The listing builds one solid part. Answer for the finished solid, in the listing's coordinates (mm). A direction names the side the tool comes from. Coordinates: 2 decimals unless noted, no trailing zeros. Loops run counter-clockwise (first coordinate to the right, second up) from the corner with the lowest first, then second, coordinate; pieces in that order, holes last. Notation, with made-up numbers: M 59,84 L 67,84 A29 cw 67,112 Z; hole C 50.5,37.25 d1. An arc over 180 degrees is marked long. Return JSON: item names as keys, results as strings. Group by question number.
1. Which of the six approach directions +Z, -Z, +X, -X, +Y, -Y give full straight-line access (tool end or side, diameter ignored) to faces 4 (the face through (21, -15, 3)), 5 (the face through (10, -20, 3)), 6 (the face through (10, 20, 3))?
2. The mould has two halves that part along Y. Classify faces 1 (the face through (9.5, -16, 3)), 2 (the face through (34.71, 20.62, 2.96)), 3 (the face through (-0.5, -17, 3)): pulls with the +Y half, pulls with the -Y half, needs draft (parallel to the pull), parting line crosses it, or undercut.
3. Straight lines are drawn through the part: L1, parallel to Y at x = 20, z = 5.05; L2, parallel to Y at x = 8, z = 3.3; L3, parallel to Y at x = -6, z = 3.9. For each, find the intervals that lie inside material, in ascending order. Write a range as from..to.
4. Section B-B (x = 13) is taken. Write down the section's boundary in (y, z).
5. Section C-C (x = -20) is taken. Write down the section's boundary in (y, z), then the cut area to 3 significant figures.
6. Given P1, Ø1.8, axis at x = 8, z = 3, coming from the +Y side; P2, Ø1.8, axis at x = 18, z = 4.5, coming from the -Y side; P3, Ø1, axis at y = -16, z = 4.5, coming from the +X side; P4, Ø3, axis at x = 13, y = 4.5, coming from the -Z side, each flat-ended and moving along its own axis, determine where each tip first touches the part or whether it passes through.
7. Section D-D (y = -8.5) is taken. Write down the section's boundary in (x, z), then the cut area to 3 significant figures.
8. Section A-A (y = 3) is taken. Write down the section's boundary in (x, z), then the cut area to 3 significant figures.
```python
from build123d import *

# Parameters (mm, degrees)
BOSS_EXTRUDE1_DEPTH = 6
SKETCH4_W           = 3
SKETCH4_H           = 3
CUT_EXTRUDE2_DEPTH  = 32
FILLET1_R           = 1
SKETCH6_W           = 53
SKETCH6_H           = 14
CUT_EXTRUDE4_DEPTH  = 44.989657875


with BuildPart() as part:
    # Sketch1 → Boss-Extrude1 (new body)
    with BuildSketch(Plane(origin=(0, 0, 0), x_dir=(0, 1, 0), z_dir=(0, 0, 1))):
        with BuildLine():
            Line((-15, -9.5), (-17, -9.5))
            ThreePointArc((-17, -9.5), (-17.707106781, -9.792893219), (-18, -10.5))
            Line((-18, -10.5), (-18, -27.5))
            Line((-18, -27.5), (-18, -37.5))
            Line((-18, -37.5), (-21.5, -37.5))
            ThreePointArc((-21.5, -37.5), (-21.959572515, -37.196959649), (-21.862068966, -36.655172414))
            ThreePointArc((-21.862068966, -36.655172414), (-20.630927937, -34.737628825), (-20.2, -32.5))
            Line((-20.2, -32.5), (-20.2, -27.5))
            Line((-20.2, -27.5), (-21.7, -27.5))
            ThreePointArc((-21.7, -27.5), (-22.120181053, -27.271012699), (-22.155497604, -26.793791532))
            Line((-22.155497604, -26.793791532), (-20.712038328, -23.6053083))
            ThreePointArc((-20.712038328, -23.6053083), (-20.180035378, -21.993620083), (-20, -20.305972812))
            Line((-20, -20.305972812), (-20, -9.5))
            Line((-20, -9.5), (-20, 0.5))
            Line((-20, 0.5), (-15, 0.5))
            Line((-15, 0.5), (-15, 32.5))
            Line((-15, 32.5), (15, 32.5))
            Line((15, 32.5), (15, 0.5))
            Line((15, 0.5), (20, 0.5))
            Line((20, 0.5), (20, -9.5))
            Line((20, -9.5), (20, -20.305972812))
            ThreePointArc((20, -20.305972812), (20.180035378, -21.993620083), (20.712038328, -23.6053083))
            Line((20.712038328, -23.6053083), (22.155497604, -26.793791532))
            ThreePointArc((22.155497604, -26.793791532), (22.120181053, -27.271012699), (21.7, -27.5))
            Line((21.7, -27.5), (20.2, -27.5))
            Line((20.2, -27.5), (20.2, -32.5))
            ThreePointArc((20.2, -32.5), (20.630927937, -34.737628825), (21.862068966, -36.655172414))
            ThreePointArc((21.862068966, -36.655172414), (21.959572515, -37.196959649), (21.5, -37.5))
            Line((21.5, -37.5), (18, -37.5))
            Line((18, -37.5), (18, -27.5))
            Line((18, -27.5), (18, -10.5))
            ThreePointArc((18, -10.5), (17.707106781, -9.792893219), (17, -9.5))
            Line((17, -9.5), (15, -9.5))
            Line((15, -9.5), (15, -32.5))
            Line((15, -32.5), (-15, -32.5))
            Line((-15, -32.5), (-15, -9.5))
        make_face()
    extrude(amount=BOSS_EXTRUDE1_DEPTH)

    # Sketch4 → Cut-Extrude2 (cut)
    with BuildSketch(Plane(origin=(-32.5, 0, 0), x_dir=(0, -1, 0), z_dir=(-1, 0, 0))):
        with Locations((-13.5, 4.5)):
            Rectangle(SKETCH4_W, SKETCH4_H)
        with Locations((13.5, 4.5)):
            Rectangle(SKETCH4_W, SKETCH4_H)
    extrude(amount=-CUT_EXTRUDE2_DEPTH, mode=Mode.SUBTRACT)

    # Fillet1
    fillet1_edges = [part.edges().sort_by_distance(p)[0] for p in [
        (-32.5, 0, 6),
        (-32.5, -15, 1.5),
        (-32.5, 15, 1.5),
        (-32.5, 13.5, 3),
        (-32.5, 12, 4.5),
        (-32.5, -12, 4.5),
        (-32.5, -13.5, 3),
        (-32.5, 0, 0),
    ]]
    fillet(fillet1_edges, radius=FILLET1_R)

    # Sketch6 → Cut-Extrude4 (cut, through all)
    with BuildSketch(Plane.XY.offset(6)):
        Rectangle(SKETCH6_W, SKETCH6_H)
    extrude(amount=-CUT_EXTRUDE4_DEPTH, mode=Mode.SUBTRACT)


solid = part.part
```
Worked out:
{
 "1": {"face 4": "+Z, -Z, +X", "face 5": "+Z, -Z, -X, -Y", "face 6": "+Z, -Z, -X, +Y"},
 "2": {"face 1": "undercut", "face 2": "pulls with the +Y half", "face 3": "needs draft"},
 "3": {"L1": "-20..-18, -15..-7, 7..15, 18..20", "L2": "-20..-7, 7..20", "L3": "-12..-7, 7..12"},
 "4": {"outline": "M -20,0 L -18,0 L -18,6 L -20,6 Z; M -15,0 L -7,0 L -7,6 L -15,6 Z; M 7,0 L 15,0 L 15,6 L 7,6 Z; M 18,0 L 20,0 L 20,6 L 18,6 Z"},
 "5": {"outline": "M -15,0 L -7,0 L -7,6 L -12,6 L -12,3 L -15,3 Z; M 7,0 L 15,0 L 15,3 L 12,3 L 12,6 L 7,6 Z", "area": "78.0 mm^2"},
 "6": {"P1": "y = 20", "P2": "y = -20", "P3": "x = 9.5", "P4": "through"},
 "7": {"outline": "M -32.5,1 A1 ccw -31.5,0 L 32.5,0 L 32.5,6 L -31.5,6 A1 ccw -32.5,5 Z", "area": "390 mm^2"},
 "8": {"outline": "M -32.5,1 A1 ccw -31.5,0 L -26.5,0 L -26.5,6 L -31.5,6 A1 ccw -32.5,5 Z; M 26.5,0 L 32.5,0 L 32.5,6 L 26.5,6 Z", "area": "71.6 mm^2"}
}
